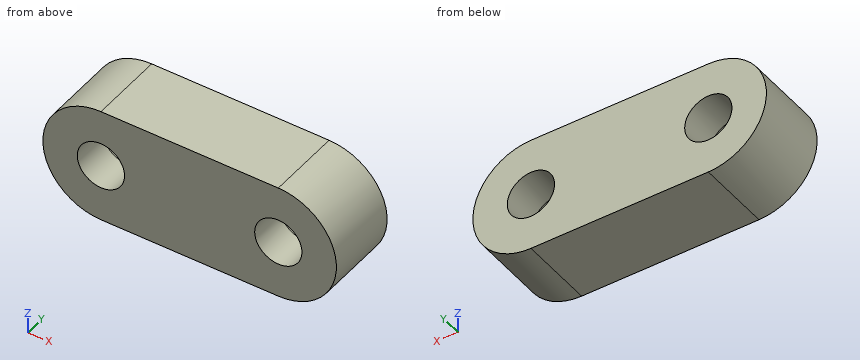
```python
from build123d import *

# Parameters (mm, degrees)
F0_R     = 4.0005
F1_DEPTH = 6.35


with BuildPart() as f1:
    # F0 (on Front) → F1 (new body, symmetric)
    with BuildSketch(Plane.XZ):
        with BuildLine():
            Line((0, -9.8298), (0, 0))
            Line((0, 0), (0, 9.8298))
            Line((0, 9.8298), (-15.0114, 9.8298))
            ThreePointArc((-15.0114, 9.8298), (-24.8412, 0), (-15.0114, -9.8298))
            Line((-15.0114, -9.8298), (0, -9.8298))
        make_face()
        with Locations((-15.0114, 0)):
            Circle(F0_R, mode=Mode.SUBTRACT)
        with BuildLine():
            Line((0, 9.8298), (0, 0))
            Line((0, 0), (0, -9.8298))
            Line((0, -9.8298), (15.0114, -9.8298))
            ThreePointArc((15.0114, -9.8298), (24.8412, 0), (15.0114, 9.8298))
            Line((15.0114, 9.8298), (0, 9.8298))
        make_face()
        with BuildLine():
            ThreePointArc((19.0119, 0), (15.0114, -4.0005), (11.0109, 0))
            ThreePointArc((11.0109, 0), (15.0114, 4.0005), (19.0119, 0))
        make_face(mode=Mode.SUBTRACT)
    extrude(amount=F1_DEPTH, both=True)


solid = f1.part
```
Check sheet for the modelled part. Datum: model origin and axes. Units: mm. Give positions to 0.01 mm unless a question says otherwise; leave off trailing zeros. Order: outer loops, then holes, each group sorted by start corner. A loop starts at its lowest first (then second) coordinate and runs counter-clockwise, first axis right, second up. Notation, with made-up numbers: (41.25, -9.75) -> (87.25, -9.75) arc R22 cw to (87.25, -2.75) -> close; hole circle Ø7 at (81, 48.5). An arc over 180 degrees is marked (long way). Use CSV: the item, a comma, the result in double quotes. Start each with the question number.
1) Sectioned sample at D-D, the plane z = 3.25. Record the boundary of the cut face in (x, y).
2) Sectioned sample at C-C, the plane x = 12.5. Record the boundary of the cut face in (y, z).
3) Material ranges on line 1 (X direction, y = -4, z = 1.25); line 2 (X direction, y = 3.5, z = -3); line 3 (Z direction, x = -13, y = -0.25), recorded low to high. Write a range as from..to.
4) Sectioned sample at B-B, the plane y = 2.5. Record the boundary of the cut face in (x, z).
5) Sectioned sample at A-A, the plane z = 0. Record the boundary of the cut face in (x, y).
6) Go/stop test with flat-tipped pins: P1, Ø2, axis at y = 1, z = 5.5, coming from the +X side; P2, Ø7, axis at x = -15.01, z = 0, coming from the +Y side; P3, Ø2, axis at y = 1.5, z = 3.5, coming from the -X side. Record where each tip stops, or that it passes through.
Recorded:
1,outline,"(-24.29, -6.35) -> (-17.34, -6.35) -> (-17.34, 6.35) -> (-24.29, 6.35) -> close; (-12.68, -6.35) -> (12.68, -6.35) -> (12.68, 6.35) -> (-12.68, 6.35) -> close; (17.34, -6.35) -> (24.29, -6.35) -> (24.29, 6.35) -> (17.34, 6.35) -> close"
2,outline,"(-6.35, -9.83) -> (6.35, -9.83) -> (6.35, -3.11) -> (-6.35, -3.11) -> close; (-6.35, 3.11) -> (6.35, 3.11) -> (6.35, 9.83) -> (-6.35, 9.83) -> close"
3,line 1,"-24.76..-18.81, -11.21..11.21, 18.81..24.76"
3,line 2,"-24.37..-17.66, -12.36..12.36, 17.66..24.37"
3,line 3,"-9.83..-3.46, 3.46..9.83"
4,outline,"(-15.01, -9.83) -> (15.01, -9.83) arc R9.83 ccw to (15.01, 9.83) -> (-15.01, 9.83) arc R9.83 ccw to start; hole circle Ø8 at (-15.01, 0); hole circle Ø8 at (15.01, 0)"
5,outline,"(-24.84, -6.35) -> (-19.01, -6.35) -> (-19.01, 6.35) -> (-24.84, 6.35) -> close; (-11.01, -6.35) -> (11.01, -6.35) -> (11.01, 6.35) -> (-11.01, 6.35) -> close; (19.01, -6.35) -> (24.84, -6.35) -> (24.84, 6.35) -> (19.01, 6.35) -> close"
6,P1,"x = 23.75"
6,P2,"through"
6,P3,"x = -24.52"
